The model under review builds one solid part; all positions refer to its coordinate system, in mm. A direction names the side the tool comes from. Give positions to 0.01 mm unless a question says otherwise; leave off trailing zeros. Order: outer loops, then holes, each group sorted by start corner. A loop starts at its lowest first (then second) coordinate and runs counter-clockwise, first axis right, second up. Notation, with made-up numbers: (32.25, -3) - (57.25, -3) arc R16 cw to (57.25, 27) - close; hole circle Ø8 at (6, -10). An arc over 180 degrees is marked (long way). Use CSV: the item, a comma, the result in double quotes. Start each with the question number.
1. Draft analysis for pull direction Z (two halves, no side actions). For faces 4 (the flat face through (13.308, -13, 0)), 5 (the flat face through (44.56, -6.26, -27.75)), 6 (the flat face through (48, -12.7, 0)), state which applies: released by +Z, released by -Z, zero draft, split by the parting line, or undercut.
2. Machinability: for faces 1 (the flat face through (8, -25.4, -8)), 2 (the flat face through (45.56, -6.26, 27.5)), 3 (the flat face through (11, -13, 3.671)), which of the approach directions +Z, -Z, +X, -X, +Y, -Y give a long, thin tool a straight path to every point of the face, cutting with its end or side? Answer none if there is none.
3. For pin 1 (2.5 mm diameter, centred on x = 10, y = -14.5, fed in from -Z); pin 2 (10 mm diameter, centred on x = 80.5, y = -54, fed in from +Z); pin 3 (1 mm diameter, centred on x = 41, z = -15, fed in from -Y); pin 4 (6 mm diameter, centred on y = -85, z = 22.5, fed in from +X), all flat-tipped, find the tip position at first contact; note any pin that passes through.
4. Take a section at A-A, the plane x = 0. State the section outline as (y, z) points (3 decimals).
5. Take a section at B-B, the plane y = -56.5. State the section outline as (x, z) points (3 decimals), then the cut area to 3 significant figures.
6. Take a section at C-C, the plane z = 16. State the section outline as (x, y) points.
7. Take a section at D-D, the plane x = 76.2. State the section outline as (y, z) points (3 decimals).
8. To check wall thickness, follow line 1 (Z direction, x = 76.2, y = -74) (3 decimals); line 2 (Y direction, x = 36, z = -23); line 3 (Y direction, x = 11.5, z = 10). State the ranges of each line that lie inside material, in increasing order. Write a range as [from, to].
```python
from build123d import *

# Parameters (mm, degrees)
F1_DEPTH = 25.4
F2_DEPTH = 12.7
F0_R     = 9.525
F3_DEPTH = 94.98793


with BuildPart() as f1:
    # F0 (on Front) → F1 (new body)
    with BuildSketch(Plane.XZ):
        with BuildLine():
            ThreePointArc((9.239379, -36.65417), (29.817356, -23.234017), (37.800718, 0))
            ThreePointArc((37.800718, 0), (29.817356, 23.234017), (9.239379, 36.65417))
            ThreePointArc((9.239379, 36.65417), (-37.800718, 0), (9.239379, -36.65417))
        make_face()
        with BuildLine():
            ThreePointArc((-8.789045, 3.671282), (0, 9.525), (8.789045, 3.671282))
            Line((8.789045, 3.671282), (13.308408, 3.671282))
            Line((13.308408, 3.671282), (13.308408, -3.671282))
            Line((13.308408, -3.671282), (8.789045, -3.671282))
            ThreePointArc((8.789045, -3.671282), (0, -9.525), (-8.789045, -3.671282))
            Line((-8.789045, -3.671282), (-13.308408, -3.671282))
            Line((-13.308408, -3.671282), (-13.308408, 3.671282))
            Line((-13.308408, 3.671282), (-8.789045, 3.671282))
        make_face(mode=Mode.SUBTRACT)
        with BuildLine():
            ThreePointArc((-8.789045, -3.671282), (-9.525, 0), (-8.789045, 3.671282))
            Line((-8.789045, 3.671282), (-13.308408, 3.671282))
            Line((-13.308408, 3.671282), (-13.308408, -3.671282))
            Line((-13.308408, -3.671282), (-8.789045, -3.671282))
        make_face()
    extrude(amount=F1_DEPTH)

    # F0 (on Front) → F2 (join)
    with BuildSketch(Plane.XZ):
        with BuildLine():
            ThreePointArc((9.239379, 36.65417), (29.817356, 23.234017), (37.800718, 0))
            ThreePointArc((37.800718, 0), (29.817356, -23.234017), (9.239379, -36.65417))
            Line((9.239379, -36.65417), (80.886979, -18.594032))
            ThreePointArc((80.886979, -18.594032), (57.024344, 0), (80.886979, 18.594032))
            Line((80.886979, 18.594032), (9.239379, 36.65417))
        make_face()
    extrude(amount=F2_DEPTH)

    # F0 (on Front) → F3 (join)
    with BuildSketch(Plane.XZ):
        with BuildLine():
            ThreePointArc((95.375656, 0), (91.325834, 11.786219), (80.886979, 18.594032))
            ThreePointArc((80.886979, 18.594032), (57.024344, 0), (80.886979, -18.594032))
            ThreePointArc((80.886979, -18.594032), (91.325834, -11.786219), (95.375656, 0))
        make_face()
        with Locations((76.2, 0)):
            Circle(F0_R, mode=Mode.SUBTRACT)
    extrude(amount=F3_DEPTH)


solid = f1.part
```
Determined:
1,face 4,"undercut"
1,face 5,"released by -Z"
1,face 6,"zero draft"
2,face 1,"+Z, -Z, -X, -Y"
2,face 2,"+Z, +X, +Y, -Y"
2,face 3,"+Y, -Y"
3,pin 1,"stops at z = -36.77"
3,pin 2,"stops at z = 19.18"
3,pin 3,"stops at y = -12.7"
3,pin 4,"passes through"
4,outline,"(-25.4, -37.801) - (0, -37.801) - (0, -9.525) - (-25.4, -9.525) - close; (-25.4, 9.525) - (0, 9.525) - (0, 37.801) - (-25.4, 37.801) - close"
5,outline,"(80.887, -18.594) arc R19.176 ccw to (95.376, 0) arc R19.176 ccw to (80.887, 18.594) arc R19.176 ccw (long way) to start; hole circle Ø19.05 at (76.2, 0)"
5,area,"870 mm²"
6,outline,"(-34.25, -25.4) - (34.25, -25.4) - (34.25, -12.7) - (65.63, -12.7) - (65.63, -94.99) - (86.77, -94.99) - (86.77, 0) - (-34.25, 0) - close"
7,outline,"(-94.988, -19.176) - (-12.7, -19.176) - (-12.7, -19.775) - (0, -19.775) - (0, -9.525) - (-94.988, -9.525) - close; (-94.988, 9.525) - (0, 9.525) - (0, 19.775) - (-12.7, 19.775) - (-12.7, 19.176) - (-94.988, 19.176) - close"
8,line 1,"z = [-19.176, -9.525], [9.525, 19.176]"
8,line 2,"y = [-12.7, 0]"
8,line 3,"y = [-25.4, 0]"
